Build history of the part. All positions in model axes, mm. A direction names the side the tool comes from. Round coordinates to 2 decimals unless told otherwise and drop trailing zeros. Loops run counter-clockwise (first coordinate to the right, second up) from the corner with the lowest first, then second, coordinate; pieces in that order, holes last.
from build123d import *

# Parameters (mm, degrees)
F4_DEPTH       = 6
F9_DEPTH       = 4.251
F10_R          = 1.9
F11_DEPTH      = 1.2
F13_DEPTH      = 8.501
F13_DEPTH_BACK = 8.501
F15_R          = 1.3
F16_DEPTH      = 1.2


# Not quite as in the source:
# - a pattern or mirror of a feature is missing from the dataset's text; its kind, count and spacing are read off the source's solid


with BuildPart() as f2:
    # F1 (on Front) → F2 (revolve)
    with BuildSketch(Plane.XZ):
        Polygon((7.3, 37.5), (7.3, 16.4), (8.5, 16.4), (8.5, 37.9970562748), (4.9970562748, 41.5), (0, 41.5), (0, 40.3), (4.5, 40.3), align=None)
    revolve(axis=Axis((0, 0, 13.2), (0, 0, -1)))

    # F3 (on face) → F4 (join)
    with BuildSketch(Plane(origin=(0, 0, 16.4), x_dir=(1, 0, 0), z_dir=(0, 0, -1))):
        with BuildLine():
            Line((7.1477269114, -4.6), (12, -4.6))
            ThreePointArc((12, -4.6), (16.6, 0), (12, 4.6))
            Line((12, 4.6), (7.1477269114, 4.6))
            ThreePointArc((7.1477269114, 4.6), (8.5, 0), (7.1477269114, -4.6))
        make_face()
    f4 = extrude(amount=-F4_DEPTH)

    # F4_copies: F4 across plane
    add(f4.mirror(Plane(origin=(0, 0, 0), x_dir=(0, 0, -1), z_dir=(-1, 0, 0))))

    # F7 (on Front) → F8 (revolve, cut)
    with BuildSketch(Plane.XZ):
        Polygon((8.5, 22.4), (10.6, 20.3), (16.6, 20.3), (16.6, 22.4), align=None)
    revolve(axis=Axis((0, 0, 13.2), (0, 0, -1)), mode=Mode.SUBTRACT)

    # F6 (on offset) → F9 (cut, through all)
    with BuildSketch(Plane(origin=(0, 0, 17.6), x_dir=(1, 0, 0), z_dir=(0, 0, -1))):
        Polygon((12, -3.4063665882), (14.95, -1.7031832941), (14.95, 1.7031832941), (12, 3.4063665882), (9.05, 1.7031832941), (9.05, -1.7031832941), align=None)
    f9 = extrude(amount=-F9_DEPTH, mode=Mode.SUBTRACT)

    # F9_copies: F9 across plane
    add(f9.mirror(Plane(origin=(0, 0, 0), x_dir=(0, 0, -1), z_dir=(-1, 0, 0))), mode=Mode.SUBTRACT)

    # F10 (on face) → F11 (cut, through all)
    with BuildSketch(Plane(origin=(0, 0, 16.4), x_dir=(1, 0, 0), z_dir=(0, 0, -1))):
        with Locations((12, 0)):
            Circle(F10_R)
    f11 = extrude(amount=-F11_DEPTH, mode=Mode.SUBTRACT)

    # F11_copies: F11 across plane
    add(f11.mirror(Plane(origin=(0, 0, 0), x_dir=(0, 0, -1), z_dir=(-1, 0, 0))), mode=Mode.SUBTRACT)

    # F12 (on Front) → F13 (cut, two sides)
    with BuildSketch(Plane.XZ) as f13_sk:
        Polygon((-4.75, 32.0470562748), (-4.75, 18.8), (4.75, 18.8), (4.75, 32.0470562748), (0, 36.7970562748), align=None)
    extrude(amount=-F13_DEPTH, mode=Mode.SUBTRACT)
    extrude(f13_sk.sketch, amount=F13_DEPTH_BACK, mode=Mode.SUBTRACT)

    # F15 (on face) → F16 (cut, through all)
    with BuildSketch(Plane.XY.offset(41.5)):
        Circle(F15_R)
    extrude(amount=-F16_DEPTH, mode=Mode.SUBTRACT)


solid = f2.part
(1) Which spindle directions (+Z, -Z, +X, -X, +Y, -Y) get a long thin tool onto all of the face, cutting with end or side? Do faces 1 (the face through (-13.5, -2.54, 18.93)), 2 (the face through (1.1, -1.1, 40.3)), 3 (the face through (-4.75, -6, 26)). Say none if no direction does.
Responses:
face 1: +Z
face 2: -Z
face 3: +Y, -Y
(2) Slice it at B-B on x = -13. List the corners of the cut face in (y, z), plus the area to 3 significant figures.
Responses:
outline: (-4.49, 16.4) - (-1.62, 16.4) - (-1.62, 17.6) - (-2.83, 17.6) - (-2.83, 20.3) - (-4.49, 20.3) - close; (1.62, 16.4) - (4.49, 16.4) - (4.49, 20.3) - (2.83, 20.3) - (2.83, 17.6) - (1.62, 17.6) - close
area: 15.9 mm2
(3) Slice it at C-C on y = 0. Count the separate pieces of the cut face and the enclosed holes in it, plus the area to 3 significant figures.
Responses:
separate pieces: 4
enclosed holes: 0
area: 94.4 mm2
(4) Slice it at A-A on z = 25. List the corners of the cut face in (x, y).
Responses:
outline: (-4.75, -7.05) - (-4.75, -5.54) arc R7.3 cw to (-4.75, 5.54) - (-4.75, 7.05) arc R8.5 ccw to start; (4.75, -7.05) arc R8.5 ccw to (4.75, 7.05) - (4.75, 5.54) arc R7.3 cw to (4.75, -5.54) - close
(5) Pull direction Y, two halves, no side cores. Call faces 4 (the face through (10.5, 2.54, 19.16)), 5 (the face through (-8.49, -0.37, 29.75)), 6 (the face through (13.5, -2.54, 18.93)), 7 (the face through (2.408, -7.329, 34.389)): +Y half, -Y half, draft (parallel to the pull), parting line (faces both ways), or undercut.
Responses:
face 4: undercut
face 5: parting line
face 6: undercut
face 7: draft
(6) Probe line 1 (X direction, y = 0, z = 16.95); line 2 (X direction, y = 0, z = 30.75); line 3 (Y direction, x = 12, z = 16.85). List the from-to ranges inside material, lowest first.
Responses:
line 1: x = -16.6 to -13.9, -10.1 to -7.3, 7.3 to 10.1, 13.9 to 16.6
line 2: x = -8.5 to -7.3, 7.3 to 8.5
line 3: y = -4.6 to -1.9, 1.9 to 4.6
(7) Pin check, flat tips, straight feed: P1, Ø4.5, axis at x = 0, y = 2, coming from the -Z side; P2, Ø6, axis at y = -4.5, z = 25, coming from the +X side; P3, Ø2.5, axis at x = 0, y = 7.5, coming from the +Z side. Stop position of each tip, or through.
Responses:
P1: stops at z = 40.3
P2: stops at x = 8.37
P3: stops at z = 40.25
(8) Slice it at D-D on z = 34.5. List the corners of the cut face in (x, y), plus the area to 3 significant figures.
Responses:
outline: (-2.3, -8.18) - (-2.3, -6.93) arc R7.3 cw to (-2.3, 6.93) - (-2.3, 8.18) arc R8.5 ccw to start; (2.3, -8.18) arc R8.5 ccw to (2.3, 8.18) - (2.3, 6.93) arc R7.3 cw to (2.3, -6.93) - close
area: 48.4 mm2
